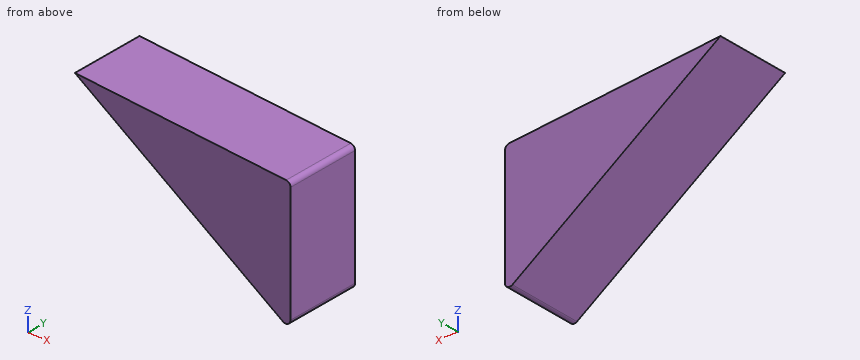
Autodesk Inventor part; units mm, degrees
ref_plane "YZ Plane" through (0, 0, 0) normal (1, 0, 0) x (0, 1, 0)
ref_plane "XZ Plane" through (0, 0, 0) normal (0, 1, 0) x (-1, 0, 0)
ref_plane "XY Plane" through (0, 0, 0) normal (0, 0, 1) x (1, 0, 0)
sketch "Sketch1" plane through (0, 0, 0) normal (0, 1, 0) x (-1, 0, 0)
  line L0 (0, 0) -> (90, 0)
  line L1 (90, 0) -> (0, -62)
  line L2 (0, -62) -> (0, 0)
  line L3 (90, 0) -> (0, -8)
  dimension "d8" = 90
  dimension "d9" = 62
  dimension "d10" = 54
extrude "Extrusion1" add sketch "Sketch1" along normal blind 32 contours L1 L2 L3
fillet "Fillet3" radius 2 2 edges at (0, 16, -8) (0, 16, -62)
properties part number "ramp"
Verification items for the finished model (mm, model axes). Give positions to 0.01 mm unless a question says otherwise; leave off trailing zeros. Order: outer loops, then holes, each group sorted by start corner. A loop starts at its lowest first (then second) coordinate and runs counter-clockwise, first axis right, second up. Notation, with made-up numbers: M -20.5,87.5 L 38.5,87.5 A12 cw 38.5,96.5 Z; hole C 58.25,0.25 d3. An arc over 180 degrees is marked long. Return JSON: item names as keys, results as strings. Group by question number.
1) Go/stop test with flat-tipped pins: pin 1 Ø1.5 at (y, z) = (15, -13) entering from -X; pin 2 Ø5 at (x, y) = (-46.5, 24) entering from -Z; pin 3 Ø3 at (x, y) = (-68.5, 24.5) entering from -Z. Record where each tip stops, or that it passes through.
2) Section check B-B on z = -26.5. Record the cut outline in (x, y).
3) Section check A-A on y = 29. Record the cut outline in (x, z).
4) Section check C-C on x = -8.5. Record the cut outline in (y, z), and give its area (3 significant figures).
5) Scan lines: line 1 (X direction, y = 23, z = -55); line 2 (X direction, y = 20, z = -47.5); line 3 (Z direction, x = -34.5, y = 11.5). Record each from-to range of solid material in increasing order.
Answer block:
{
 "1": {"pin 1": "stops at x = -72.22", "pin 2": "stops at z = -31.69", "pin 3": "stops at z = -15.84"},
 "2": {"outline": "M -51.53,0 L 0,0 L 0,32 L -51.53,32 Z"},
 "3": {"outline": "M -90,0 L -3.13,-59.84 A2 ccw 0,-58.19 L 0,-9.83 A2 ccw -1.82,-7.84 Z"},
 "4": {"outline": "M 0,-56.14 L 32,-56.14 L 32,-7.24 L 0,-7.24 Z", "area": "1,560 mm^2"},
 "5": {"line 1": "x = -10.16 to 0", "line 2": "x = -21.05 to 0", "line 3": "z = -38.23 to -4.93"}
}
